Could you check a few things on this drawing? It's one solid part, dimensions in mm from its lowest x, y, z. A direction names the side the tool comes from. Round coordinates to 2 decimals unless told otherwise and drop trailing zeros. Loops run counter-clockwise (first coordinate to the right, second up) from the corner with the lowest first, then second, coordinate; pieces in that order, holes last. Notation, with made-up numbers: M -32,-38 L 7,-38 A23 cw 7,-4 Z; hole C -22,49.5 d6. An arc over 180 degrees is marked long. Answer as CSV lines item,"result".
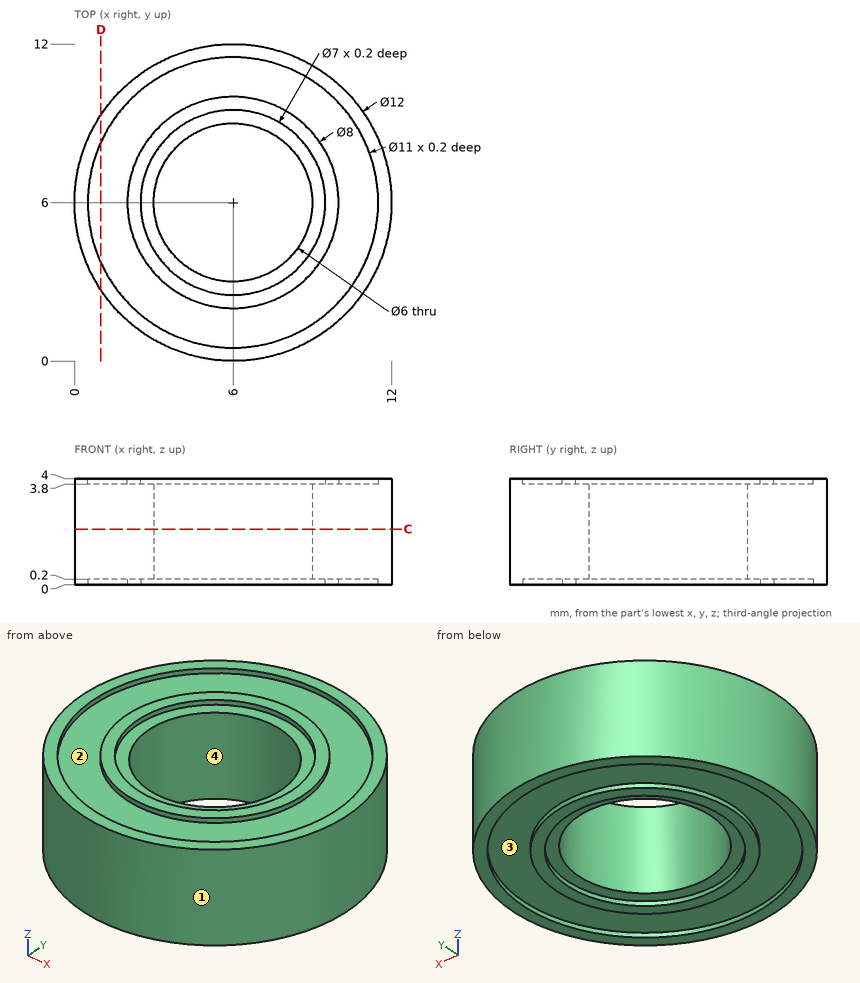
Item 1: If we section it at D-D on x = 1: Write out the boundary of the cut face in (y, z), then the cut area to 3 significant figures.
Output:
outline,"M 2.68,0 L 3.71,0 L 3.71,0.2 L 8.29,0.2 L 8.29,0 L 9.32,0 L 9.32,4 L 8.29,4 L 8.29,3.8 L 3.71,3.8 L 3.71,4 L 2.68,4 Z"
area,"24.7 mm2"
Item 2: Will these pins go through, and if not, where does the flat tip stop? pin 1 (5.5 mm diameter, centred on x = 6, y = 6, fed in from -Z); pin 2 (1.5 mm diameter, centred on x = 3, z = 3.5, fed in from +Y).
Output:
pin 1,"passes through"
pin 2,"stops at y = 11.56"
Item 3: We'd pull the mould along X, two halves only. Please class the marked faces 1 and 2: released by +X, released by -X, zero draft, split by the parting line, or undercut.
Output:
face 1,"split by the parting line"
face 2,"undercut"
Item 4: If we section it at C-C on z = 2.1: Write out the boundary of the cut face in (x, y).
Output:
outline,"C 6,6 d12; hole C 6,6 d6"
Item 5: If I drill on line 1 along Y through (x, z) = (6, 3.9); line 2 along Y through (x, z) = (6, 1.9); line 3 along Z through (x, y) = (1, 5.5), over which ranges is the centre line in solid material (lowest first)? Write a range as from..to.
Output:
line 1,"y = 0..0.5, 2..2.5, 9.5..10, 11.5..12"
line 2,"y = 0..3, 9..12"
line 3,"z = 0.2..3.8"
Item 6: On a 3-axis mill with a long thin cutter (end or side, diameter ignored), from which of +Z, -Z, +X, -X, +Y, -Y can I reach the whole of each face in a straight line? I mean the marked faces 3 and 4. Say none if no direction works.
Output:
face 3,"-Z"
face 4,"+Z, -Z"
